```python
from build123d import *

# Parameters (mm, degrees)
SKETCH_1_W          = 100
SKETCH_1_H          = 10
EXTRUDE_1_DEPTH     = 3
SKETCH_2_R          = 1.25
CUT_EXTRUDE_1_DEPTH = 51.338851795
CHAMFER_1_SIZE      = 1


with BuildPart() as part:
    # 草图1 → 凸台-拉伸1 (new body)
    with BuildSketch(Plane(origin=(0, 0, 0), x_dir=(0, 0, -1), z_dir=(1, 0, 0))):
        Rectangle(SKETCH_1_W, SKETCH_1_H)
    extrude(amount=EXTRUDE_1_DEPTH)

    # 草图2 → 切除-拉伸1 (cut, through all)
    with BuildSketch(Plane(origin=(3, 0, 0), x_dir=(0, 0, -1), z_dir=(1, 0, 0))):
        with Locations((-45, 0)):
            Circle(SKETCH_2_R)
        with Locations((45, 0)):
            Circle(SKETCH_2_R)
    extrude(amount=-CUT_EXTRUDE_1_DEPTH, mode=Mode.SUBTRACT)

    # 倒角1
    chamfer_1_edges = [part.edges().sort_by_distance(p)[0] for p in [
        (1.5, 5, 50),
        (1.5, 5, -50),
        (1.5, -5, -50),
        (1.5, -5, 50),
    ]]
    chamfer(chamfer_1_edges, length=CHAMFER_1_SIZE)


solid = part.part
```
Verification items for the finished model (mm, model axes). Give positions to 0.01 mm unless a question says otherwise; leave off trailing zeros. Order: outer loops, then holes, each group sorted by start corner. A loop starts at its lowest first (then second) coordinate and runs counter-clockwise, first axis right, second up. Notation, with made-up numbers: M 79.25,41 L 119.25,41 A36 cw 119.25,75 Z; hole C 72,-24 d7. An arc over 180 degrees is marked long. Return JSON: item names as keys, results as strings. Group by question number.
1) Go/stop test with flat-tipped pins: pin 1 Ø3 at (y, z) = (0, -45) entering from -X; pin 2 Ø1.5 at (y, z) = (0, 45) entering from -X. Record where each tip stops, or that it passes through.
2) Section check A-A on z = -45. Record the cut outline in (x, y), and give its area (3 significant figures).
3) Scan lines: line 1 (Y direction, x = 0.95, z = 45); line 2 (Z direction, x = 1.1, y = 1); line 3 (Z direction, x = 1.8, y = 0.5). Record each from-to range of solid material in increasing order.
4) Mould release check, pull along Y, two halves, no side actions. Record for faces 1 (the face through (1, 0, 50)), 2 (the face through (1, 5, 1)), 3 (the face through (1.52, 0.05, -43.75)): pulls with the +Y half, pulls with the -Y half, needs draft (parallel to the pull), parting line crosses it, or undercut.
5) Section check B-B on y = 0. Record the cut outline in (x, z), and give its area (3 significant figures).
Answer block:
{
 "1": {"pin 1": "stops at x = 0", "pin 2": "passes through"},
 "2": {"outline": "M 0,-5 L 3,-5 L 3,-1.25 L 0,-1.25 Z; M 0,1.25 L 3,1.25 L 3,5 L 0,5 Z", "area": "22.5 mm^2"},
 "3": {"line 1": "y = -5 to -1.25, 1.25 to 5", "line 2": "z = -50 to -45.75, -44.25 to 44.25, 45.75 to 50", "line 3": "z = -50 to -46.15, -43.85 to 43.85, 46.15 to 50"},
 "4": {"face 1": "needs draft", "face 2": "pulls with the +Y half", "face 3": "undercut"},
 "5": {"outline": "M 0,-50 L 3,-50 L 3,-46.25 L 0,-46.25 Z; M 0,-43.75 L 3,-43.75 L 3,43.75 L 0,43.75 Z; M 0,46.25 L 3,46.25 L 3,50 L 0,50 Z", "area": "285 mm^2"}
}
